```python
from build123d import *

# Parameters (mm, degrees)
F0_W        = 76.2
F0_H        = 152.4
F1_DEPTH    = 6.35
F2_DEPTH    = 25.4
F3_DEPTH    = 50.8
F4_C1_SIZE2 = 12.7
F4_C1_SIZE  = 12.26424744
F4_C2_SIZE2 = 12.7
F4_C2_SIZE  = 12.26424744
F4_C3_SIZE2 = 12.26424744
F4_C3_SIZE  = 12.7
F4_C4_SIZE2 = 12.7
F4_C4_SIZE  = 12.26424744
F4_C5_SIZE2 = 12.26424744
F4_C5_SIZE  = 12.7
F4_C6_SIZE2 = 12.26424744
F4_C6_SIZE  = 12.7
F4_C7_SIZE2 = 12.26424744
F4_C7_SIZE  = 12.7
F4_C8_SIZE2 = 12.26424744
F4_C8_SIZE  = 12.7
F5_R        = 6.34999


# Not quite as in the source:
# - a fillet or chamfer is up to 0.001 mm smaller than in the source, because OpenCascade refuses the exact size


with BuildPart() as f1:
    # F0 (on Top) → F1 (new body)
    with BuildSketch(Plane.XY):
        with Locations((0, -69.85)):
            Rectangle(F0_W, F0_H)
        Polygon((-31.75, -31.75), (-31.75, 0), (0, 0), (31.75, 0), (31.75, -107.95), (31.75, -139.7), (0, -139.7), (-31.75, -139.7), align=None, mode=Mode.SUBTRACT)
    extrude(amount=F1_DEPTH)

    # F0 (on Top) → F2 (join)
    with BuildSketch(Plane.XY):
        with BuildLine():
            Line((31.75, 0), (0, 0))
            Line((0, 0), (0, -19.05))
            ThreePointArc((0, -19.05), (-3.7197438789, -28.0302561211), (-12.7, -31.75))
            Line((-12.7, -31.75), (-31.75, -31.75))
            Line((-31.75, -31.75), (-31.75, -139.7))
            Line((-31.75, -139.7), (0, -139.7))
            Line((0, -139.7), (0, -120.65))
            ThreePointArc((0, -120.65), (3.7197438789, -111.6697438789), (12.7, -107.95))
            Line((12.7, -107.95), (31.75, -107.95))
            Line((31.75, -107.95), (31.75, 0))
        make_face()
    extrude(amount=F2_DEPTH)

    # F0 (on Top) → F3 (join)
    with BuildSketch(Plane.XY):
        with BuildLine():
            Line((0, 0), (-31.75, 0))
            Line((-31.75, 0), (-31.75, -31.75))
            Line((-31.75, -31.75), (-12.7, -31.75))
            ThreePointArc((-12.7, -31.75), (-3.7197438789, -28.0302561211), (0, -19.05))
            Line((0, -19.05), (0, 0))
        make_face()
        with BuildLine():
            Line((31.75, -139.7), (31.75, -107.95))
            Line((31.75, -107.95), (12.7, -107.95))
            ThreePointArc((12.7, -107.95), (3.7197438789, -111.6697438789), (0, -120.65))
            Line((0, -120.65), (0, -139.7))
            Line((0, -139.7), (31.75, -139.7))
        make_face()
    extrude(amount=F3_DEPTH)

    # F4: chamfer of 12.7 x 12.26424744 on 8 edges, made by hand

    # F4_c1
    f4_c1_edges = [f1.edges().sort_by_distance(p)[0] for p in [
        (-15.875, -139.7, 25.4),
    ]]
    f4_c1_side = f1.faces().sort_by_distance((-15.875, -139.7, 25.1547150512))[0]
    chamfer(f4_c1_edges, length=F4_C1_SIZE, length2=F4_C1_SIZE2, reference=f4_c1_side)

    # F4_c2
    f4_c2_edges = [f1.edges().sort_by_distance(p)[0] for p in [
        (15.875, -139.7, 50.8),
    ]]
    f4_c2_side = f1.faces().sort_by_distance((15.875, -139.7, 50.5547150512))[0]
    chamfer(f4_c2_edges, length=F4_C2_SIZE, length2=F4_C2_SIZE2, reference=f4_c2_side)

    # F4_c3
    f4_c3_edges = [f1.edges().sort_by_distance(p)[0] for p in [
        (31.75, -117.475, 50.8),
    ]]
    f4_c3_side = f1.faces().sort_by_distance((31.75, -117.475, 50.5547150512))[0]
    chamfer(f4_c3_edges, length=F4_C3_SIZE, length2=F4_C3_SIZE2, reference=f4_c3_side)

    # F4_c4
    f4_c4_edges = [f1.edges().sort_by_distance(p)[0] for p in [
        (15.875, 0, 25.4),
    ]]
    f4_c4_side = f1.faces().sort_by_distance((15.875, 0, 25.1547150512))[0]
    chamfer(f4_c4_edges, length=F4_C4_SIZE, length2=F4_C4_SIZE2, reference=f4_c4_side)

    # F4_c5
    f4_c5_edges = [f1.edges().sort_by_distance(p)[0] for p in [
        (-31.75, -79.375, 25.4),
    ]]
    f4_c5_side = f1.faces().sort_by_distance((-31.5047150512, -79.375, 25.4))[0]
    chamfer(f4_c5_edges, length=F4_C5_SIZE, length2=F4_C5_SIZE2, reference=f4_c5_side)

    # F4_c6
    f4_c6_edges = [f1.edges().sort_by_distance(p)[0] for p in [
        (31.75, -60.325, 25.4),
    ]]
    f4_c6_side = f1.faces().sort_by_distance((31.5047150512, -60.325, 25.4))[0]
    chamfer(f4_c6_edges, length=F4_C6_SIZE, length2=F4_C6_SIZE2, reference=f4_c6_side)

    # F4_c7
    f4_c7_edges = [f1.edges().sort_by_distance(p)[0] for p in [
        (-15.875, 0, 50.8),
    ]]
    f4_c7_side = f1.faces().sort_by_distance((-15.875, 0, 50.5547150512))[0]
    chamfer(f4_c7_edges, length=F4_C7_SIZE, length2=F4_C7_SIZE2, reference=f4_c7_side)

    # F4_c8
    f4_c8_edges = [f1.edges().sort_by_distance(p)[0] for p in [
        (-31.75, -22.00712372, 50.8),
    ]]
    f4_c8_side = f1.faces().sort_by_distance((-31.5047150512, -22.00712372, 50.8))[0]
    chamfer(f4_c8_edges, length=F4_C8_SIZE, length2=F4_C8_SIZE2, reference=f4_c8_side)

    # F5 (radius 6.35 in the source; OpenCascade refuses exactly that, so slightly less here)
    f5_edges = [f1.edges().sort_by_distance(p)[0] for p in [
        (38.1, -69.85, 6.35),
        (0, 6.35, 6.35),
        (-38.1, -69.85, 6.35),
        (0, -146.05, 6.35),
    ]]
    fillet(f5_edges, radius=F5_R)


solid = f1.part
```
The listing builds one solid part. Answer for the finished solid, in the listing's coordinates (mm). A direction names the side the tool comes from. Coordinates: 2 decimals unless noted, no trailing zeros. Write each loop counter-clockwise with the first axis right and the second up, starting at its lowest first coordinate (ties: lowest second). Pieces come first, ordered by that corner, then holes. Notation, with made-up numbers: (83.5, -5) - (121.5, -5) arc R34 cw to (121.5, 32) - close; hole circle Ø6 at (-9, 17). An arc over 180 degrees is marked (long way). One line per item, written item: value.
1) Each of these flat-tipped pins is pushed along its axis until it touches: pin 1 Ø21 at (x, z) = (-21, 27) entering from -Y; pin 2 Ø5 at (x, z) = (-7, 43.5) entering from -Y; pin 3 Ø3 at (x, z) = (26, 35) entering from +Y. Where does it stop, or does it pass through?
Geometry check:
pin 1: stops at y = -136.22
pin 2: stops at y = -31.34
pin 3: stops at y = -107.95
2) A tool of negligible diameter and unlimited length cuts with its end or side. For faces 1 (the flat face through (25.49, -54.73, 19.18)), 2 (the flat face through (-12.569, -133.261, 19.354)), 3 (the flat face through (31.75, -102, 11)), from which of +Z, -Z, +X, -X, +Y, -Y can it reach the whole face along a straight path? Write none if from no direction.
Geometry check:
face 1: +Z, +X, +Y
face 2: +Z, -X, -Y
face 3: +Z, +X, +Y, -Y
3) Find section D-D (z = 11). Give the vertices of the cut face in (x, y), and give its area (3 significant figures).
Geometry check:
outline: (-31.75, -139.7) - (31.75, -139.7) - (31.75, 0) - (-31.75, 0) - close
area: 8,870 mm2
4) Consider line 1 along Z through (x, y) = (11.5, -30); line 2 along X through (y, z) = (-97.5, 10.5); line 3 along X through (y, z) = (-130.5, 22.5). Determine where each line is inside the solid, lowest interval first. Write a range as from..to.
Geometry check:
line 1: z = 0..25.4
line 2: x = -31.75..31.75
line 3: x = 0..31.75
5) Find section A-A (z = 29.5). Give the vertices of the cut face in (x, y), and give its area (3 significant figures).
Geometry check:
outline: (-31.75, -31.75) - (-12.7, -31.75) arc R12.7 ccw to (0, -19.05) - (0, 0) - (-31.75, 0) - close; (0, -139.7) - (31.75, -139.7) - (31.75, -107.95) - (12.7, -107.95) arc R12.7 ccw to (0, -120.65) - close
area: 1,950 mm2
